from build123d import *

# Parameters (mm, degrees)
BOSS_EXTRUDE1_DEPTH = 20
SKETCH3_R           = 2.1
CUT_EXTRUDE1_DEPTH  = 43.842719799
SKETCH4_R           = 7.5
BOSS_EXTRUDE2_DEPTH = 7
SKETCH5_R           = 8
BOSS_EXTRUDE3_DEPTH = 3
SKETCH6_R           = 7.5
BOSS_EXTRUDE4_DEPTH = 7
SKETCH7_R           = 6
CUT_EXTRUDE2_DEPTH  = 77.839573439
FILLET1_R           = 1
CHAMFER1_SIZE       = 0.5
CHAMFER2_SIZE       = 2
FILLET2_R           = 0.5


with BuildPart() as part:
    # Sketch1 → Boss-Extrude1 (new body)
    with BuildSketch(Plane.XY):
        with BuildLine():
            Line((38.3, 10.745623604), (38.3, 9.881410941))
            Line((38.3, 9.881410941), (38.3, 5.394343623))
            Line((38.3, 5.394343623), (38.3, -11.605656377))
            ThreePointArc((38.3, -11.605656377), (38.885786438, -13.01986994), (40.3, -13.605656377))
            Line((40.3, -13.605656377), (51.3, -13.605656377))
            Line((51.3, -13.605656377), (56.3, -13.605656377))
            ThreePointArc((56.3, -13.605656377), (57.714213562, -13.01986994), (58.3, -11.605656377))
            Line((58.3, -11.605656377), (58.3, 7.881410941))
            ThreePointArc((58.3, 7.881410941), (57.714213562, 9.295624503), (56.3, 9.881410941))
            Line((56.3, 9.881410941), (45.3, 9.881410941))
            ThreePointArc((45.3, 9.881410941), (43.885786438, 10.467197379), (43.3, 11.881410941))
            Line((43.3, 11.881410941), (43.3, 31.710978016))
            ThreePointArc((43.3, 31.710978016), (42.714213562, 33.125191579), (41.3, 33.710978016))
            Line((41.3, 33.710978016), (39.3, 33.710978016))
            ThreePointArc((39.3, 33.710978016), (38.592893219, 33.418084798), (38.3, 32.710978016))
            Line((38.3, 32.710978016), (38.3, 28.215588568))
            Line((38.3, 28.215588568), (38.3, 27.353495632))
            Line((38.3, 27.353495632), (38.3, 24.630195866))
            ThreePointArc((38.3, 24.630195866), (37.780173169, 23.37522288), (36.525200183, 22.855396049))
            Line((36.525200183, 22.855396049), (35.6108, 22.855396049))
            ThreePointArc((35.6108, 22.855396049), (34.355826885, 23.375222934), (33.836, 24.630196049))
            Line((33.836, 24.630196049), (33.836, 28.448))
            ThreePointArc((33.836, 28.448), (33.634196572, 28.935196572), (33.147, 29.137))
            Line((33.147, 29.137), (32.664287242, 29.137))
            ThreePointArc((32.664287242, 29.137), (32.400617966, 29.084552836), (32.177090071, 28.935195973))
            Line((32.177090071, 28.935195973), (27.33900161, 24.097095612))
            ThreePointArc((27.33900161, 24.097095612), (26.352731832, 22.621035632), (26.0064, 20.879905136))
            Line((26.0064, 20.879905136), (26.0064, 17.220094864))
            ThreePointArc((26.0064, 17.220094864), (26.352731832, 15.478964368), (27.33900161, 14.002904388))
            Line((27.33900161, 14.002904388), (32.090366071, 9.25152824))
            ThreePointArc((32.090366071, 9.25152824), (32.409953896, 9.037986056), (32.786933649, 8.963))
            Line((32.786933649, 8.963), (33.060275787, 8.963))
            ThreePointArc((33.060275787, 8.963), (33.608795638, 9.190204362), (33.836, 9.738724213))
            Line((33.836, 9.738724213), (33.836, 13.469803585))
            ThreePointArc((33.836, 13.469803585), (34.355826992, 14.724776959), (35.610800366, 15.244603951))
            Line((35.610800366, 15.244603951), (36.5252, 15.244603951))
            ThreePointArc((36.5252, 15.244603951), (37.780173115, 14.724777066), (38.3, 13.469803951))
            Line((38.3, 13.469803951), (38.3, 10.745623604))
        make_face()
    extrude(amount=-BOSS_EXTRUDE1_DEPTH)

    # Sketch3 → Cut-Extrude1 (cut, through all)
    with BuildSketch(Plane(origin=(43.3, 0, 0), x_dir=(0, 0, -1), z_dir=(1, 0, 0))):
        with Locations((5, 18.710978016)):
            Circle(SKETCH3_R)
        with Locations(Location((15, 18.710978016, 0), (0, 0, 314.769611651))):
            Circle(SKETCH3_R)
    extrude(amount=-CUT_EXTRUDE1_DEPTH, mode=Mode.SUBTRACT)

    # Sketch4 → Boss-Extrude2 (add)
    with BuildSketch(Plane(origin=(0, 0, -20), x_dir=(-1, 0, 0), z_dir=(0, 0, -1))):
        with Locations(Location((-48.3, -1.862122718, 0), (0, 0, 180))):
            Circle(SKETCH4_R)
    extrude(amount=BOSS_EXTRUDE2_DEPTH)

    # Sketch5 → Boss-Extrude3 (add)
    with BuildSketch(Plane(origin=(0, 0, -27), x_dir=(-1, 0, 0), z_dir=(0, 0, -1))):
        with Locations((-48.3, -1.862122718)):
            Circle(SKETCH5_R)
    extrude(amount=BOSS_EXTRUDE3_DEPTH)

    # Sketch6 → Boss-Extrude4 (add)
    with BuildSketch(Plane(origin=(0, 0, -30), x_dir=(-1, 0, 0), z_dir=(0, 0, -1))):
        with Locations(Location((-48.3, -1.862122718, 0), (0, 0, 180))):
            Circle(SKETCH6_R)
    extrude(amount=BOSS_EXTRUDE4_DEPTH)

    # Sketch7 → Cut-Extrude2 (cut, through all)
    with BuildSketch(Plane(origin=(0, 0, -37), x_dir=(-1, 0, 0), z_dir=(0, 0, -1))):
        with Locations((-48.3, -1.862122718)):
            Circle(SKETCH7_R)
    extrude(amount=-CUT_EXTRUDE2_DEPTH, mode=Mode.SUBTRACT)

    # Fillet1
    fillet1_edges = [part.edges().sort_by_distance(p)[0] for p in [
        (40.8, -1.862122718, -20),
    ]]
    fillet(fillet1_edges, radius=FILLET1_R)

    # Chamfer1
    chamfer1_edges = [part.edges().sort_by_distance(p)[0] for p in [
        (40.8, -1.862122718, -27),
        (40.8, -1.862122718, -30),
    ]]
    chamfer(chamfer1_edges, length=CHAMFER1_SIZE - 0.0001)  # a hair under: the kernel refuses the full size

    # Chamfer2
    chamfer2_edges = [part.edges().sort_by_distance(p)[0] for p in [
        (54.3, -1.862122718, 0),
    ]]
    chamfer(chamfer2_edges, length=CHAMFER2_SIZE)

    # Fillet2
    fillet2_edges = [part.edges().sort_by_distance(p)[0] for p in [
        (40.8, -1.862122718, -37),
        (54.3, -1.862122718, -37),
    ]]
    fillet(fillet2_edges, radius=FILLET2_R)


solid = part.part
Geometry: final body of the model. Coordinates: model frame, mm. A direction names the side the tool comes from. Coordinates: 2 decimals unless noted, no trailing zeros. Write each loop counter-clockwise with the first axis right and the second up, starting at its lowest first coordinate (ties: lowest second). Pieces come first, ordered by that corner, then holes. Notation, with made-up numbers: (34, -0.75) - (92, -0.75) arc R18 cw to (92, 25.25) - close; hole circle Ø4 at (34, -34.5). An arc over 180 degrees is marked (long way). Return JSON: item names as keys, results as strings.
Item 1: Pull-direction query (Z, two-part tool) for faces 4 (the face through (42, 10, 0)), 5 (the face through (40.67, 0.54, -28.48)), 6 (the face through (55.454, -4.115, -23.712)); classes: +Z half, -Z half, draft (parallel to the pull), parting line (faces both ways), or undercut.
Completed:
{"face 4": "+Z half", "face 5": "draft", "face 6": "undercut"}
Item 2: Reachability of faces 1 (the face through (51, 9.881, -10)), 2 (the face through (33.836, 12, -10)), 3 (the face through (37.794, 23.389, -9.86)) from +Z, -Z, +X, -X, +Y, -Y: full face, straight path, thin tool, end or side. Return the list, or none.
Completed:
{"face 1": "+Z, -Z, +X, +Y", "face 2": "+Z, -Z, -Y", "face 3": "+Z, -Z, +Y"}
Item 3: Section query D-D (z = -24). Output: boundary loops of the cut face in (x, y), and give its area (3 significant figures).
Completed:
{"outline": "circle Ø15 at (48.3, -1.86); hole circle Ø12 at (48.3, -1.86)", "area": "63.6 mm2"}
Item 4: Pin query (flat end, axial travel): pin 1 Ø7 at (x, y) = (48.3, -1.86) entering from -Z; pin 2 Ø6 at (x, z) = (35.5, -7) entering from +Y; pin 3 Ø5 at (x, y) = (48, -6) entering from +Z; pin 4 Ø10 at (y, z) = (-2.5, -5.5) entering from -X. Return the tip coordinate at first contact, or that it passes through.
Completed:
{"pin 1": "passes through", "pin 2": "stops at y = 33.31", "pin 3": "stops at z = -1.35", "pin 4": "stops at x = 38.3"}
Item 5: Section query C-C (x = 28). Output: boundary loops of the cut face in (y, z), and give its area (3 significant figures).
Completed:
{"outline": "(13.34, -20) - (24.76, -20) - (24.76, 0) - (13.34, 0) - close; hole circle Ø4.2 at (18.71, -15); hole circle Ø4.2 at (18.71, -5)", "area": "201 mm2"}
Item 6: Section query B-B (z = -15). Count the separate pieces of the cut face and the enclosed holes in it, and give its area (3 significant figures).
Completed:
{"separate pieces": "2", "enclosed holes": "1", "area": "553 mm2"}
Item 7: Line query: L1, parallel to Y at x = 48.3, z = -19; L2, parallel to Y at x = 33, z = -5; L3, parallel to X at y = -9, z = -13. Output: solid intervals per line, ascending.
Completed:
{"L1": "y = -13.61 to -7.86, 4.14 to 9.88", "L2": "y = 8.96 to 16.61, 20.81 to 29.14", "L3": "x = 38.3 to 58.3"}
